from build123d import *

# Parameters (mm, degrees)
SKETCH1_W           = 70
SKETCH1_H           = 50
SKETCH1_R           = 2
BOSS_EXTRUDE1_DEPTH = 3
SKETCH2_W           = 52.5
SKETCH2_H           = 15.87
BOSS_EXTRUDE2_DEPTH = 4.83


with BuildPart() as part:
    # Sketch1 → Boss-Extrude1 (new body)
    with BuildSketch(Plane.XY.offset(-23)):
        with Locations((-14.828582329, -15.804770786)):
            Rectangle(SKETCH1_W, SKETCH1_H)
        with Locations((15.171417671, -35.804770786)):
            Circle(SKETCH1_R, mode=Mode.SUBTRACT)
        with Locations((-44.828582329, -35.804770786)):
            Circle(SKETCH1_R, mode=Mode.SUBTRACT)
        with Locations((-44.828582329, 4.195229214)):
            Circle(SKETCH1_R, mode=Mode.SUBTRACT)
        with Locations((15.171417671, 4.195229214)):
            Circle(SKETCH1_R, mode=Mode.SUBTRACT)
    extrude(amount=-BOSS_EXTRUDE1_DEPTH)

    # Sketch2 → Boss-Extrude2 (add)
    with BuildSketch(Plane(origin=(0, 0, -26), x_dir=(-1, 0, 0), z_dir=(0, 0, -1))):
        with Locations((16.078582329, -2.869770786)):
            Rectangle(SKETCH2_W, SKETCH2_H)
    extrude(amount=BOSS_EXTRUDE2_DEPTH)


solid = part.part
Work out the finished part from the listing and answer in its coordinate system (mm). A direction names the side the tool comes from. Give positions to 0.01 mm unless a question says otherwise; leave off trailing zeros. Order: outer loops, then holes, each group sorted by start corner. A loop starts at its lowest first (then second) coordinate and runs counter-clockwise, first axis right, second up. Notation, with made-up numbers: (12.25, 25) -> (71.25, 25) arc R20 cw to (71.25, 44) -> close; hole circle Ø4 at (-27, 87.5). An arc over 180 degrees is marked (long way). Answer as a JSON object with one key per item and string values. Group by question number.
1. Section C-C on x = -23 is taken. Determine the outline of the cut face in (y, z).
2. Section D-D on z = -28 is taken. Determine the outline of the cut face in (x, y).
3. The mould has two halves that part along Y. Classify faces 1 (the flat face through (-49.829, -16, -24)), 2 (the flat face through (-16, -10.805, -28)), 3 (the flat face through (-15, 9.195, -24)), 4 (the cylindrical face through (13.584, 2.978, -24.479)): released by +Y, released by -Y, zero draft, split by the parting line, or undercut.
4. Flat-ended cylindrical pins translate along their axes: pin 1 Ø2.5 at (x, z) = (-8, -28.5) entering from +Y; pin 2 Ø4 at (y, z) = (1, -29) entering from +X; pin 3 Ø12 at (x, y) = (-42, -22) entering from -Z. Find the tip coordinate at first contact, or state that the pin passes through.
5. Section B-B on y = -4 is taken. Determine the outline of the cut face in (x, z), plus the area to 3 significant figures.
6. A tool of negligible diameter and unlimited length cuts with its end or side. For faces 5 (the flat face through (10.171, -3, -28)), 6 (the flat face through (-16, 5.065, -28)), 7 (the cylindrical face through (14.91, -33.82, -24.48)), 8 (the flat face through (-42.329, -3, -28)), from which of +Z, -Z, +X, -X, +Y, -Y can it reach the whole face along a straight path? Write none if from no direction.
7. Section A-A on x = -44.5 is taken. Determine the outline of the cut face in (y, z), plus the area to 3 significant figures.
8. Consider line 1 along X through (y, z) = (4, -24.75); line 2 along Y through (x, z) = (-43.5, -23.5); line 3 along Z through (x, y) = (-29, -18.5). Determine where each line is inside the solid, lowest interval first. Write a range as [from, to].
Result sheet:
{
 "1": {"outline": "(-40.8, -26) -> (-10.8, -26) -> (-10.8, -30.83) -> (5.07, -30.83) -> (5.07, -26) -> (9.2, -26) -> (9.2, -23) -> (-40.8, -23) -> close"},
 "2": {"outline": "(-42.33, -10.8) -> (10.17, -10.8) -> (10.17, 5.07) -> (-42.33, 5.07) -> close"},
 "3": {"face 1": "zero draft", "face 2": "released by -Y", "face 3": "released by +Y", "face 4": "undercut"},
 "4": {"pin 1": "stops at y = 5.07", "pin 2": "stops at x = 10.17", "pin 3": "stops at z = -26"},
 "5": {"outline": "(-49.83, -26) -> (-42.33, -26) -> (-42.33, -30.83) -> (10.17, -30.83) -> (10.17, -26) -> (20.17, -26) -> (20.17, -23) -> (-49.83, -23) -> close", "area": "464 mm^2"},
 "6": {"face 5": "-Z, +X, +Y, -Y", "face 6": "-Z, +X, -X, +Y", "face 7": "+Z, -Z", "face 8": "-Z, -X, +Y, -Y"},
 "7": {"outline": "(-40.8, -26) -> (-37.78, -26) -> (-37.78, -23) -> (-40.8, -23) -> close; (-33.83, -26) -> (2.22, -26) -> (2.22, -23) -> (-33.83, -23) -> close; (6.17, -26) -> (9.2, -26) -> (9.2, -23) -> (6.17, -23) -> close", "area": "126 mm^2"},
 "8": {"line 1": "x = [-49.83, -46.82], [-42.84, 13.18], [17.16, 20.17]", "line 2": "y = [-40.8, -37.3], [-34.31, 2.7], [5.69, 9.2]", "line 3": "z = [-26, -23]"}
}
